from build123d import *

# Parameters (mm, degrees)
SKETCH_1_R               = 2.5
SKETCH_1_W               = 3
SKETCH_1_H               = 5
EXTRUDE_2_DEPTH          = 26
CUT_EXTRUDE_3_REACH      = 151.57
SKETCH_5_W               = 18
SKETCH_5_H               = 14
CUT_EXTRUDE_5_DEPTH      = 180.392084627
CUT_EXTRUDE_5_DEPTH_BACK = 22
SKETCH_7_R               = 1.5
SKETCH_8_W               = 17
SKETCH_8_H               = 17
CUT_EXTRUDE_6_DEPTH      = 190.681647041
SKETCH_9_W               = 18
SKETCH_9_H               = 14
CUT_EXTRUDE_7_DEPTH      = 15
FILLET_1_R               = 3
FILLET_2_R               = 3
FILLET_3_R               = 3
FILLET_4_R               = 3


with BuildPart() as part:
    # 草图1 → 凸台-拉伸2 (new body)
    # profile 1 of 3: a face of its own
    with BuildSketch(Plane.XY):
        Polygon((8.838520664, 62.0602), (8.838520664, 87.0602), (44.838520664, 87.0602), (44.838520664, 10.0602), (44.838520664, 5.0602), (59.838520664, 5.0602), (59.838520664, 87.0602), (143.838520664, 87.0602), (143.838520664, 109.0602), (-6.161479336, 109.0602), (-6.161479336, 87.0602), (-6.161479336, 67.0602), (-6.161479336, 62.0602), align=None)
        with Locations(Location((52.338520664, 10.0602, 0), (0, 0, 180))):
            Circle(SKETCH_1_R, mode=Mode.SUBTRACT)
        with Locations(Location((1.338520664, 67.0602, 0), (0, 0, 180))):
            Circle(SKETCH_1_R, mode=Mode.SUBTRACT)
    # profile 2 of 3: a face of its own
    with BuildSketch(Plane.XY):
        with Locations((-7.661479336, 64.5602)):
            Rectangle(SKETCH_1_W, SKETCH_1_H)
    # profile 3 of 3: a face of its own
    with BuildSketch(Plane.XY):
        with Locations((43.338520664, 7.5602)):
            Rectangle(SKETCH_1_W, SKETCH_1_H)
    extrude(amount=EXTRUDE_2_DEPTH)

    # 草图5 → 切除-拉伸3 (cut, up to next)
    with BuildSketch(Plane.ZY.offset(-44.838520664), mode=Mode.PRIVATE) as cut_extrude_3_sk1:
        with Locations((13, 12.0602)):
            Rectangle(SKETCH_5_W, SKETCH_5_H)
    cut_extrude_3_tool1 = extrude(cut_extrude_3_sk1.sketch, amount=-CUT_EXTRUDE_3_REACH, mode=Mode.PRIVATE) & part.part
    add(cut_extrude_3_tool1.solids().sort_by_distance((44.838521, 12.0602, 13))[0], mode=Mode.SUBTRACT)

    # 草图7 → 切除-拉伸5 (cut, two sides: drawn at the far end of the back side and taken through both)
    with BuildSketch(Plane(origin=(0, 109.0602, 0), x_dir=(1, 0, 0), z_dir=(0, 1, 0)).offset(-CUT_EXTRUDE_5_DEPTH_BACK)):
        with Locations(Location((128.837370272, -13, 0), (0, 0, 270))):
            Circle(SKETCH_7_R)
        with Locations(Location((128.837370272, -8, 0), (0, 0, 270))):
            Circle(SKETCH_7_R)
        with Locations(Location((128.837370272, -18, 0), (0, 0, 270))):
            Circle(SKETCH_7_R)
    extrude(amount=CUT_EXTRUDE_5_DEPTH + CUT_EXTRUDE_5_DEPTH_BACK, mode=Mode.SUBTRACT)

    # 草图8 → 切除-拉伸6 (cut, through all)
    with BuildSketch(Plane(origin=(143.838520664, 0, 0), x_dir=(0, 0, -1), z_dir=(1, 0, 0))):
        with Locations((-13, 98.0602)):
            Rectangle(SKETCH_8_W, SKETCH_8_H)
    extrude(amount=-CUT_EXTRUDE_6_DEPTH, mode=Mode.SUBTRACT)

    # 草图9 → 切除-拉伸7 (cut)
    with BuildSketch(Plane(origin=(8.838520664, 0, 0), x_dir=(0, 0, -1), z_dir=(1, 0, 0))):
        with Locations((-13, 69.0602)):
            Rectangle(SKETCH_9_W, SKETCH_9_H)
    extrude(amount=-CUT_EXTRUDE_7_DEPTH, mode=Mode.SUBTRACT)

    # 圆角1
    fillet_1_edges = [part.edges().sort_by_distance(p)[0] for p in [
        (59.838520664, 87.0602, 13),
        (8.838520664, 87.0602, 13),
    ]]
    fillet(fillet_1_edges, radius=FILLET_1_R)

    # 圆角2
    fillet_2_edges = [part.edges().sort_by_distance(p)[0] for p in [
        (44.838520664, 87.0602, 13),
    ]]
    fillet(fillet_2_edges, radius=FILLET_2_R)

    # 圆角3
    fillet_3_edges = [part.edges().sort_by_distance(p)[0] for p in [
        (8.838520664, 62.0602, 24),
    ]]
    fillet(fillet_3_edges, radius=FILLET_3_R)

    # 圆角4
    fillet_4_edges = [part.edges().sort_by_distance(p)[0] for p in [
        (8.838520664, 62.0602, 2),
        (59.838520664, 5.0602, 24),
        (59.838520664, 5.0602, 2),
    ]]
    fillet(fillet_4_edges, radius=FILLET_4_R)


solid = part.part
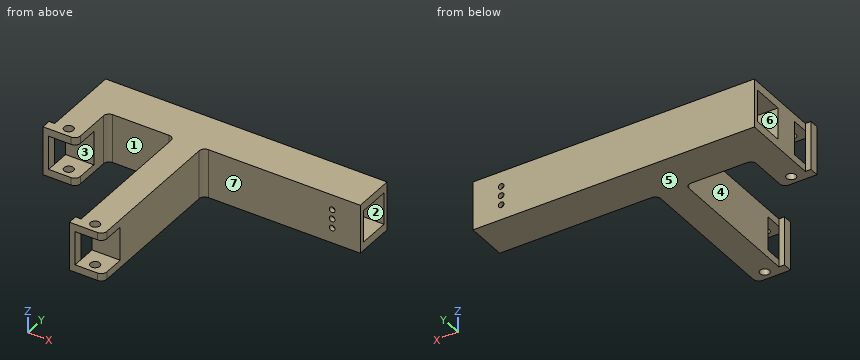
Geometry check sheet. Reference: the model listing, model coordinates, mm. Face numbers are marked on the shaded views. A direction names the side the tool comes from. Give positions to 0.01 mm unless a question says otherwise; leave off trailing zeros. Write each loop counter-clockwise with the first axis right and the second up, starting at its lowest first coordinate (ties: lowest second). Pieces come first, ordered by that corner, then holes. Notation, with made-up numbers: (1, 63) - (53, 63) arc R11 cw to (53, 77) - close; hole circle Ø8 at (56.25, 15.5). An arc over 180 degrees is marked (long way). Put each result on its own line as item: value.
1. Draft check along Y on the marked faces 5, 6 and 7. Enter one of: +Y half, -Y half, draft (parallel to the pull), parting line (faces both ways), or undercut.
Ans:
face 5: draft
face 6: undercut
face 7: -Y half
2. Sectioned sample at A-A, the plane y = 80. Enter the section's corners in (x, z).
Ans:
outline: (-6.16, 0) - (8.84, 0) - (8.84, 26) - (-6.16, 26) - close; (44.84, 0) - (59.84, 0) - (59.84, 26) - (44.84, 26) - close
3. Sectioned sample at B-B, the plane z = 13. Give the number of separate pieces and of enclosed holes in the cut face, plus the area to 3 significant figures.
Ans:
separate pieces: 6
enclosed holes: 0
area: 1,960 mm²
4. Set-up check for the marked faces 1, 2, 3 and 4: record each of +Z, -Z, +X, -X, +Y, -Y from which the full face is reachable in a straight line by a thin tool's end or side.
Ans:
face 1: +Z, -Z, -Y
face 2: +X, -X
face 3: -X, -Y
face 4: +Z, -Z
5. Thickness scan on line 1 (Y direction, x = 77, z = 19); line 2 (Y direction, x = 42, z = 7.25); line 3 (X direction, y = 63, z = 9). Record the ranges inside material, lowest first.
Ans:
line 1: y = 87.06 to 89.56, 106.56 to 109.06
line 2: y = 5.06 to 10.06, 87.06 to 89.56, 106.56 to 109.06
line 3: x = -9.16 to -6.16, 44.84 to 59.84
6. Go/stop test with flat-tipped pins: pin 1 (18.5 mm diameter, centred on x = 75.5, y = 102.5, fed in from -Z); pin 2 (8 mm diameter, centred on x = 84, z = 13, fed in from -Y); pin 3 (2 mm diameter, centred on y = 33, z = 9.5, fed in from -X); pin 4 (12 mm diameter, centred on x = 1, z = 10.5, fed in from -Y). Record where each tip stops, or that it passes through.
Ans:
pin 1: stops at z = 0
pin 2: stops at y = 87.06
pin 3: stops at x = 44.84
pin 4: stops at y = 76.06
7. Sectioned sample at C-C, the plane x = 100. Enter the section's corners in (y, z).
Ans:
outline: (87.06, 0) - (109.06, 0) - (109.06, 26) - (87.06, 26) - close; hole (89.56, 4.5) - (106.56, 4.5) - (106.56, 21.5) - (89.56, 21.5) - close
8. Sectioned sample at D-D, the plane y = 48. Enter the section's corners in (x, z).
Ans:
outline: (44.84, 0) - (59.84, 0) - (59.84, 26) - (44.84, 26) - close
